```python
from build123d import *

# Parameters (mm, degrees)
F1_DEPTH = 247.5
F3_DEPTH = 28
F4_R     = 4.25
F5_DEPTH = 25
F6_R     = 5.25
F7_DEPTH = 25
F8_R     = 5.25
F9_DEPTH = 25
F10_R    = 2
F11_R    = 0.5
F12_R    = 1


# Not quite as in the source:
# - a pattern or mirror of a feature is missing from the dataset's text; its kind, count and spacing are read off the source's solid


with BuildPart() as f1:
    # F0 (on Top) → F1 (new body, symmetric)
    with BuildSketch(Plane.XY):
        Polygon((-19.75, 3.25), (-19.75, -19.75), (-9.25, -19.75), (19.75, 9.25), (19.75, 19.75), (-3.25, 19.75), (-3.25, 16.75), (16.75, 16.75), (16.75, 10.4926406871), (-10.4926406871, -16.75), (-16.75, -16.75), (-16.75, 3.25), align=None)
    extrude(amount=F1_DEPTH, both=True)

    # F2 (on face) → F3 (cut)
    with BuildSketch(Plane.XY.offset(247.5)):
        Polygon((-10.4926406871, -16.75), (-16.75, -16.75), (-19.75, -16.75), (-19.75, -19.75), (-9.25, -19.75), (19.75, 9.25), (19.75, 19.75), (16.75, 19.75), (16.75, 16.75), (16.75, 10.4926406871), align=None)
    f3 = extrude(amount=-F3_DEPTH, mode=Mode.SUBTRACT)

    # F3_copies: F3 across plane
    add(f3.mirror(Plane(origin=(0, 0, 0), x_dir=(-1, 0, 0), z_dir=(0, 0, -1))), mode=Mode.SUBTRACT)

    # F4 (on face) → F5 (cut)
    with BuildSketch(Plane(origin=(5.25, -5.25, 0), x_dir=(0.7071067812, 0.7071067812, 0), z_dir=(0.7071067812, -0.7071067812, 0))):
        with Locations((0, 168)):
            Circle(F4_R)
        with Locations((0, -168)):
            Circle(F4_R)
        Circle(F4_R)
    extrude(amount=-F5_DEPTH, mode=Mode.SUBTRACT)

    # F6 (on face) → F7 (cut)
    with BuildSketch(Plane.YZ.offset(-16.75)):
        with Locations((-6.75, 235.5)):
            Circle(F6_R)
        with Locations((-6.75, -235.5)):
            Circle(F6_R)
    extrude(amount=-F7_DEPTH, mode=Mode.SUBTRACT)

    # F8 (on face) → F9 (cut)
    with BuildSketch(Plane.XZ.offset(-16.75)):
        with Locations((6.75, 235.5)):
            Circle(F8_R)
        with Locations((6.75, -235.5)):
            Circle(F8_R)
    extrude(amount=-F9_DEPTH, mode=Mode.SUBTRACT)

    # F10
    f10_edges = [f1.edges().sort_by_distance(p)[0] for p in [
        (-9.25, -19.75, 0),
        (19.75, 9.25, 0),
        (-18.25, -16.75, 247.5),
        (-18.25, 3.25, 247.5),
        (-3.25, 18.25, 247.5),
        (16.75, 18.25, 247.5),
        (-18.25, 3.25, -247.5),
        (-3.25, 18.25, -247.5),
        (-18.25, -16.75, -247.5),
        (16.75, 18.25, -247.5),
    ]]
    fillet(f10_edges, radius=F10_R)

    # F11
    f11_edges = [f1.edges().sort_by_distance(p)[0] for p in [
        (-10.492641, -16.75, 0),
        (16.75, 10.492641, 0),
    ]]
    fillet(f11_edges, radius=F11_R)

    # F12
    f12_edges = [f1.edges().sort_by_distance(p)[0] for p in [
        (-19.75, -19.75, 0),
        (19.75, 19.75, 0),
    ]]
    fillet(f12_edges, radius=F12_R)


solid = f1.part
```
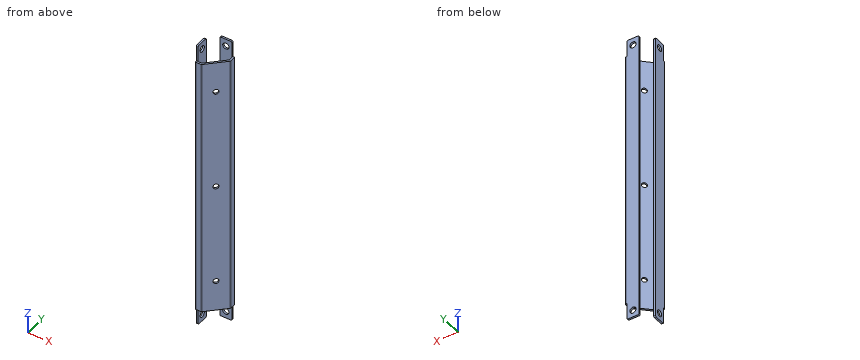
Input: part model. Units: mm. Frame: model coordinates. Give positions to 0.01 mm unless a question says otherwise; leave off trailing zeros. Order: outer loops, then holes, each group sorted by start corner. A loop starts at its lowest first (then second) coordinate and runs counter-clockwise, first axis right, second up. Notation, with made-up numbers: M 24.25,81.25 L 53.25,81.25 A9 ccw 53.25,91.25 Z; hole C 80.5,-4.5 d8. An arc over 180 degrees is marked long. Return JSON: item names as keys, results as strings.
1) Section query A-A on z = 235.5. Output: boundary loops of the cut face in (x, y).
Taken from the geometry:
{"outline": "M -19.75,-16.75 L -16.75,-16.75 L -16.75,-12 L -19.75,-12 Z; M -19.75,-1.5 L -16.75,-1.5 L -16.75,3.25 L -19.75,3.25 Z; M -3.25,16.75 L 1.5,16.75 L 1.5,19.75 L -3.25,19.75 Z; M 12,16.75 L 16.75,16.75 L 16.75,19.75 L 12,19.75 Z"}
2) Section query B-B on z = 21. Output: boundary loops of the cut face in (x, y), and give its area (3 significant figures).
Taken from the geometry:
{"outline": "M -19.75,-18.75 A1 ccw -18.75,-19.75 L -10.08,-19.75 A2 ccw -8.66,-19.16 L 19.16,8.66 A2 ccw 19.75,10.08 L 19.75,18.75 A1 ccw 18.75,19.75 L -3.25,19.75 L -3.25,16.75 L 16.75,16.75 L 16.75,10.7 A0.5 cw 16.6,10.35 L -10.35,-16.6 A0.5 cw -10.7,-16.75 L -16.75,-16.75 L -16.75,3.25 L -19.75,3.25 Z", "area": "298 mm2"}
3) Line query: L1, parallel to Z at x = 6.75, y = 17.65; L2, parallel to X at y = 18, z = -235; L3, parallel to X at y = 11, z = -51. Output: solid intervals per line, ascending. Write a range as [from, to].
Taken from the geometry:
{"L1": "z = [-247.5, -240.75], [-230.25, 230.25], [240.75, 247.5]", "L2": "x = [-3.25, 1.52], [11.98, 16.75]", "L3": "x = [16.75, 19.75]"}
4) Contact query for flat-ended pins moving along their axis: pin 1 (2 mm diameter, centred on y = -4, z = -139.5, fed in from +X); pin 2 (3 mm diameter, centred on x = -12, z = 185, fed in from +Y); pin 3 (5 mm diameter, centred on y = 13, z = -20.5, fed in from -X). Output: stop coordinate, or through.
Taken from the geometry:
{"pin 1": "stops at x = 7.5", "pin 2": "stops at y = -16.71", "pin 3": "stops at x = 16.71"}
